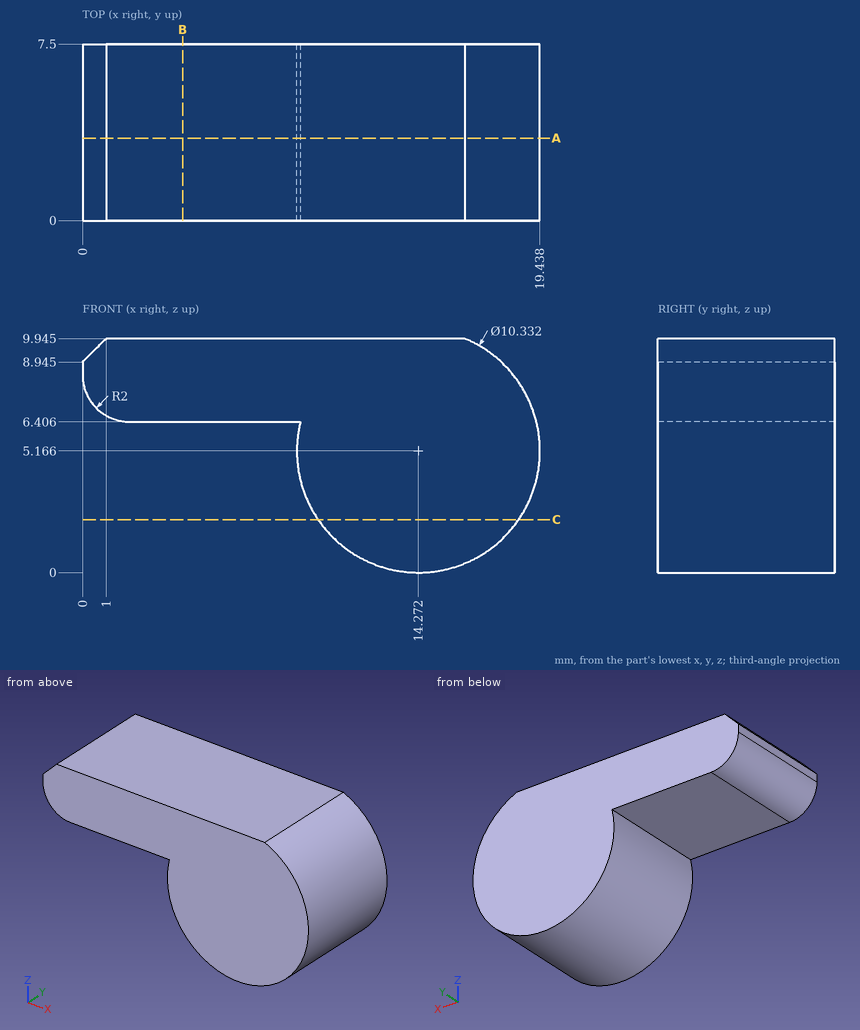
Part print with two shaded views. Sizes in mm from the minimum x, y, z corner. Round coordinates to 2 decimals unless told otherwise and drop trailing zeros. Order: outer loops, then holes, each group sorted by start corner. A loop starts at its lowest first (then second) coordinate and runs counter-clockwise, first axis right, second up. Notation, with made-up numbers: (5, 14.25) -> (35, 14.25) arc R36 ccw to (35, 48.25) -> close; hole circle Ø10 at (63.25, -28). An arc over 180 degrees is marked (long way). Write each question's results on one line, items separated by ' | '.
1. Cut at C-C (z = 2.25). Give the cut face in (x, y).
Findings below:
outline: (10.01, 0) -> (18.54, 0) -> (18.54, 7.5) -> (10.01, 7.5) -> close
2. Wall check: line 1 along Z through (x, y) = (4, 5.5) (1 decimal); line 2 along X through (y, z) = (3.75, 5) (1 decimal); line 3 along X through (y, z) = (2.75, 4) (1 decimal). Give the ranges that are in metal, low to high. Write a range as [from, to].
Findings below:
line 1: z = [6.4, 9.9] | line 2: x = [9.1, 19.4] | line 3: x = [9.2, 19.3]
3. Flat gauge pins, fed straight in: P1, Ø4, axis at y = 2, z = 1.5, coming from the +X side; P2, Ø2, axis at x = 4.5, y = 4, coming from the -Z side; P3, Ø1.5, axis at y = 3, z = 8, coming from the +X side. Where does each tip first touch, or does it go through?
Findings below:
P1: stops at x = 19.16 | P2: stops at z = 6.41 | P3: stops at x = 19
4. Cut at A-A (y = 3.5). Give the cut face in (x, z) (1 decimal).
Findings below:
outline: (0, 8.4) arc R2 ccw to (2, 6.4) -> (9.3, 6.4) arc R5.2 ccw (long way) to (16.2, 9.9) -> (1, 9.9) -> (0, 8.9) -> close
5. Cut at B-B (x = 4.25). Give the cut face in (y, z) (1 decimal).
Findings below:
outline: (0, 6.4) -> (7.5, 6.4) -> (7.5, 9.9) -> (0, 9.9) -> close
